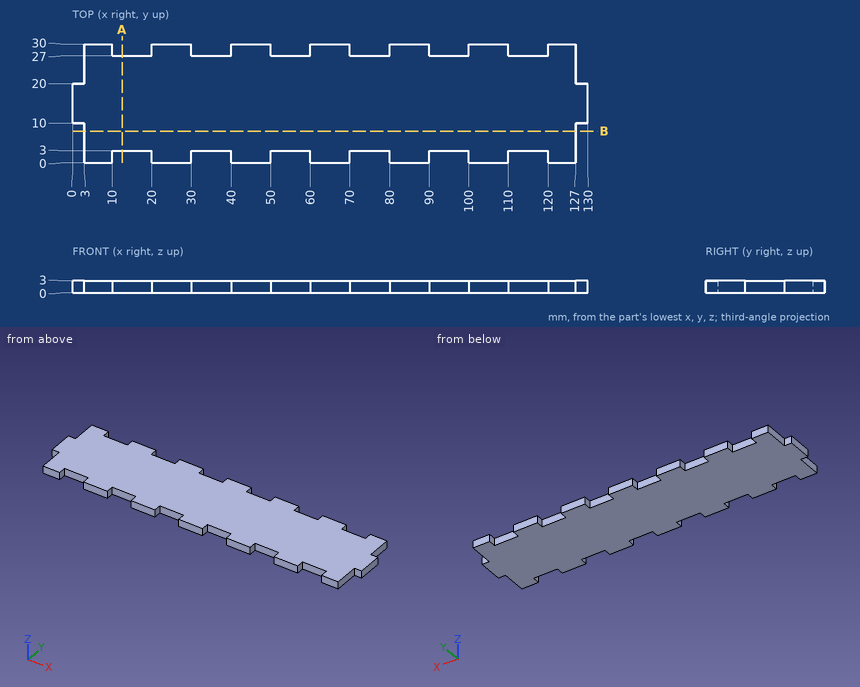
Verification items for this drawing (mm, ordinates from the low corner). Give positions to 0.01 mm unless a question says otherwise; leave off trailing zeros. Write each loop counter-clockwise with the first axis right and the second up, starting at its lowest first coordinate (ties: lowest second). Pieces come first, ordered by that corner, then holes. Notation, with made-up numbers: (61, 89.25) - (74, 89.25) arc R32 ccw to (74, 119.25) - close; hole circle Ø6 at (66, -11.75). An arc over 180 degrees is marked (long way). Answer as a JSON object with one key per item and string values. Group by question number.
1) Sectioned sample at B-B (y = 8). Record the cut outline in (x, z), then the cut area to 3 significant figures.
2) Depth check by flat-ended pin: P1, Ø0.9, axis at y = 2, z = 2, coming from the -X side; P2, Ø0.9, axis at x = 115.5, z = 2, coming from the +Y side; P3, Ø1, axis at y = 3, z = 1.5, coming from the +X side. Enter the tip coordinate at first touch or a pass-through.
3) Thickness scan on probe 1 along Y at (x, z) = (95, 1.3); probe 2 along X at (y, z) = (3.5, 1.95). Record the ranges inside material, lowest first. Write a range as from..to.
4) Sectioned sample at A-A (x = 12.5). Record the cut outline in (y, z), then the cut area to 3 significant figures.
Geometry results:
{
 "1": {"outline": "(3, 0) - (127, 0) - (127, 3) - (3, 3) - close", "area": "372 mm^2"},
 "2": {"P1": "stops at x = 3", "P2": "stops at y = 27", "P3": "stops at x = 127"},
 "3": {"probe 1": "y = 3..27", "probe 2": "x = 3..127"},
 "4": {"outline": "(3, 0) - (27, 0) - (27, 3) - (3, 3) - close", "area": "72.0 mm^2"}
}
